Part model, mm, in its own coordinate system. Face numbers are marked on the shaded views. A direction names the side the tool comes from. Coordinates: 2 decimals unless noted, no trailing zeros. Loops run counter-clockwise (first coordinate to the right, second up) from the corner with the lowest first, then second, coordinate; pieces in that order, holes last. Notation, with made-up numbers: (-5, 75.25) -> (9, 75.25) arc R20 ccw to (9, 87.25) -> close; hole circle Ø11 at (-3.5, 89). An arc over 180 degrees is marked (long way). One line per item, written item: value. Start each with the question number.
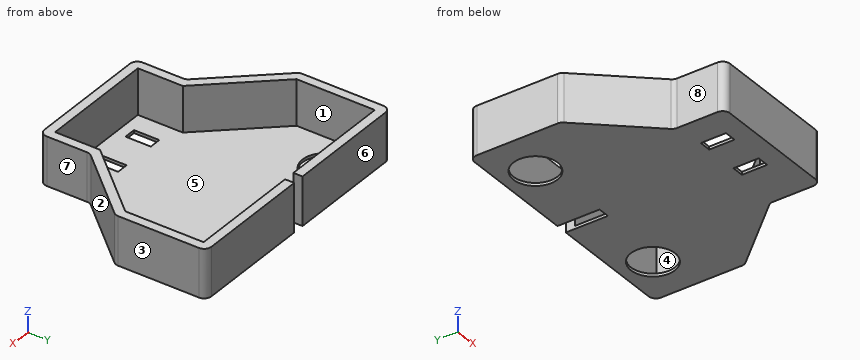
Autodesk Inventor part; units mm, degrees
ref_plane "YZ Plane" through (0, 0, 0) normal (1, 0, 0) x (0, 1, 0)
ref_plane "XZ Plane" through (0, 0, 0) normal (0, 1, 0) x (-1, 0, 0)
ref_plane "Work Plane1" through (0, 0, -5.08) normal (0, 0, 1) x (1, 0, 0)
sketch "Sketch1" plane through (0, 0, -5.08) normal (0, 0, 1) x (1, 0, 0)
  line L0 (20.772, 33.401) -> (20.772, 19.8332)
  line L1 (20.772, 33.401) -> (1.011, 33.401)
  line L2 (1.011, 33.401) -> (1.011, 27.686)
  line L3 (1.011, 27.686) -> (-1.011, 27.686)
  line L4 (-1.011, 27.686) -> (-1.011, 33.401)
  line L5 (-1.011, 33.401) -> (-20.772, 33.401)
  line L6 (-20.772, 33.401) -> (-20.772, 19.8332)
  line L7 (-20.772, 19.8332) -> (-10.033, 7.78)
  line L8 (-10.033, 7.78) -> (-10.033, 0)
  line L9 (-10.033, 0) -> (10.033, 0)
  line L10 (10.033, 0) -> (10.033, 7.78)
  line L11 (10.033, 7.78) -> (20.772, 19.8332)
  line L12 (-22.3595, 34.9885) -> (-0.5765, 34.9885)
  line L13 (-0.5765, 34.9885) -> (22.3595, 34.9885)
  line L14 (22.3595, 34.9885) -> (22.3595, 19.2286)
  line L15 (22.3595, 19.2286) -> (11.6205, 7.1754)
  line L16 (11.6205, 7.1754) -> (11.6205, -1.5875)
  line L17 (11.6205, -1.5875) -> (-11.6205, -1.5875)
  line L18 (-11.6205, -1.5875) -> (-11.6205, 7.1754)
  line L19 (-11.6205, 7.1754) -> (-22.3595, 19.2286)
  line L20 (-22.3595, 19.2286) -> (-22.3595, 34.9885)
  point P0 (0, 0)
  point P1 (0, 0)
  point P2 (0, 27.686)
  point P3 (0, 0)
  dimension "d1" = 41.544
  dimension "d2" = 19.761
  dimension "d3" = 19.761
  dimension "d6" = 20.066
  dimension "d7" = 138.3
  dimension "d8" = 138.3
  dimension "d9" = 33.401
  dimension "d10" = 5.715
  dimension "d11" = 25.621
  dimension "d12" = 1.5875
extrude "Extrusion1" add sketch "Sketch1" along normal blind 8.382
extrude "Extrusion2" add sketch "Sketch1" along normal blind 0.508 contours L0 L11 L10 L9 L8 L7 L6 L5 L4 L3 L2 L1
sketch "Sketch2" plane through (0, 0, 3.302) normal (0, 0, 1) x (1, 0, 0)
  line L0 (-22.3595, 34.9885) -> (22.3595, 34.9885) construction
  line L1 (-1.011, 27.686) -> (1.011, 27.686)
  line L2 (1.011, 27.686) -> (1.011, 34.9885)
  line L3 (1.011, 34.9885) -> (-1.011, 34.9885)
  line L4 (-1.011, 34.9885) -> (-1.011, 27.686)
  point P0 (0, 0)
extrude "Extrusion3" cut sketch "Sketch2" against normal through all
fillet "Fillet1" radius 1.27 8 edges at (-22.3595, 34.9885, -0.889) (-22.3595, 19.2286, -0.889) (-11.6205, 7.1754, -0.889) (-11.6205, -1.5875, -0.889) (11.6205, -1.5875, -0.889) (11.6205, 7.1754, -0.889) (22.3595, 19.2286, -0.889) (22.3595, 34.9885, -0.889)
sketch "Sketch4" plane through (0, 0, -5.08) normal (0, 0, -1) x (-1, 0, 0)
  circle A0 centre (-14.2442, 29.337) radius 1.8288 construction
  circle A1 centre (14.2546, 29.337) radius 1.8288 construction
  circle A2 centre (-14.2442, 29.337) radius 3.81
  circle A3 centre (14.2546, 29.337) radius 3.81
  line L0 (-1.8894, 5.6982) -> (-2.9308, 5.6982) construction
  line L1 (-2.9308, 2.3282) -> (-2.9308, 5.6982) construction
  line L2 (-2.9308, 2.3282) -> (-1.8894, 2.3282) construction
  line L3 (-1.8894, 5.6982) -> (-1.8894, 2.3282) construction
  line L4 (6.0354, 5.6982) -> (4.994, 5.6982) construction
  line L5 (4.994, 2.3282) -> (4.994, 5.6982) construction
  line L6 (4.994, 2.3282) -> (6.0354, 2.3282) construction
  line L7 (6.0354, 5.6982) -> (6.0354, 2.3282) construction
  line L8 (-1.3814, 1.8202) -> (-3.4388, 1.8202)
  line L9 (-3.4388, 1.8202) -> (-3.4388, 6.2062)
  line L10 (-3.4388, 6.2062) -> (-1.3814, 6.2062)
  line L11 (-1.3814, 6.2062) -> (-1.3814, 1.8202)
  line L12 (4.486, 6.2062) -> (6.5434, 6.2062)
  line L13 (6.5434, 6.2062) -> (6.5434, 1.8202)
  line L14 (6.5434, 1.8202) -> (4.486, 1.8202)
  line L15 (4.486, 1.8202) -> (4.486, 6.2062)
  point P0 (0, 0)
  dimension "d30" = 7.62
  dimension "d33" = 0.508
  dimension "d34" = 0.508
extrude "Extrusion4" cut sketch "Sketch4" against normal blind 25.4
equation "\"d3\" = d2"
equation "\"d8\" = d7"
properties part number "kracken Cover" material "Aluminum 6061"
1) Pull direction Y, two halves, no side cores. Call the marked faces 1, 2, 3 and 4: +Y half, -Y half, draft (parallel to the pull), parting line (faces both ways), or undercut.
2) Slice it at D-D (x = -19). Give the cut face in (y, z).
3) Slice it at B-B (y = 31). Give the cut face in (x, z), then the cut area to 3 significant figures.
4) Slice it at A-A (x = 11). Give the cut face in (y, z), then the cut area to 3 significant figures.
5) Probe line 1 (Y direction, x = 4, z = -1.75); line 2 (X direction, y = 6.5, z = -2); line 3 (X direction, y = 33.5, z = 2.25). List the from-to ranges inside material, lowest first. Write a range as from..to.
6) Tool access for the marked faces 5, 6, 7 and 8: list every direction of +Z, -Z, +X, -X, +Y, -Y with a clear straight run to the whole face (end or side of a thin tool).
7) Pin check, flat tips, straight feed: pin 1 Ø1.5 at (y, z) = (7.5, 2) entering from +X; pin 2 Ø6 at (x, y) = (14.24, 29.34) entering from +Z; pin 3 Ø4 at (y, z) = (3, 0.5) entering from +X; pin 4 Ø1.5 at (y, z) = (6.5, 2) entering from +X. Stop position of each tip, or through.
8) Slice it at C-C (z = -2.75). Give the cut face in (x, y).
Check sheet entries:
1. face 1: undercut
1. face 2: -Y half
1. face 3: draft
1. face 4: undercut
2. outline: (15.46, -5.08) -> (34.99, -5.08) -> (34.99, 3.3) -> (33.4, 3.3) -> (33.4, -4.57) -> (17.84, -4.57) -> (17.84, 3.3) -> (15.46, 3.3) -> close
3. outline: (-22.36, -5.08) -> (-17.68, -5.08) -> (-17.68, -4.57) -> (-20.77, -4.57) -> (-20.77, 3.3) -> (-22.36, 3.3) -> close; (-10.83, -5.08) -> (-1.01, -5.08) -> (-1.01, -4.57) -> (-10.83, -4.57) -> close; (1.01, -5.08) -> (10.82, -5.08) -> (10.82, -4.57) -> (1.01, -4.57) -> close; (17.67, -5.08) -> (22.36, -5.08) -> (22.36, 3.3) -> (20.77, 3.3) -> (20.77, -4.57) -> (17.67, -4.57) -> close
3. area: 39.7 mm^2
4. outline: (-1.41, -5.08) -> (27.34, -5.08) -> (27.34, -4.57) -> (8.87, -4.57) -> (8.87, 3.3) -> (-1.41, 3.3) -> close; (31.33, -5.08) -> (34.99, -5.08) -> (34.99, 3.3) -> (33.4, 3.3) -> (33.4, -4.57) -> (31.33, -4.57) -> close
4. area: 110 mm^2
5. line 1: y = -1.59..0, 33.4..34.99
5. line 2: x = -11.62..-10.03, 10.03..11.62
5. line 3: x = -22.36..-1.01, 1.01..22.36
6. face 5: +Z
6. face 6: +Z, -Z, +X, -X, +Y
6. face 7: +Z, -Z, +X, -Y
6. face 8: +Z, -Z, -X, -Y
7. pin 1: stops at x = 12.58
7. pin 2: passes through
7. pin 3: stops at x = 11.62
7. pin 4: stops at x = 11.75
8. outline: (-22.36, 19.71) arc R1.27 ccw to (-22.04, 18.87) -> (-11.94, 7.54) arc R1.27 cw to (-11.62, 6.69) -> (-11.62, -0.32) arc R1.27 ccw to (-10.35, -1.59) -> (10.35, -1.59) arc R1.27 ccw to (11.62, -0.32) -> (11.62, 6.69) arc R1.27 cw to (11.94, 7.54) -> (22.04, 18.87) arc R1.27 ccw to (22.36, 19.71) -> (22.36, 33.72) arc R1.27 ccw to (21.09, 34.99) -> (1.01, 34.99) -> (1.01, 33.4) -> (20.77, 33.4) -> (20.77, 19.83) -> (10.03, 7.78) -> (10.03, 0) -> (-10.03, 0) -> (-10.03, 7.78) -> (-20.77, 19.83) -> (-20.77, 33.4) -> (-1.01, 33.4) -> (-1.01, 34.99) -> (-21.09, 34.99) arc R1.27 ccw to (-22.36, 33.72) -> close
